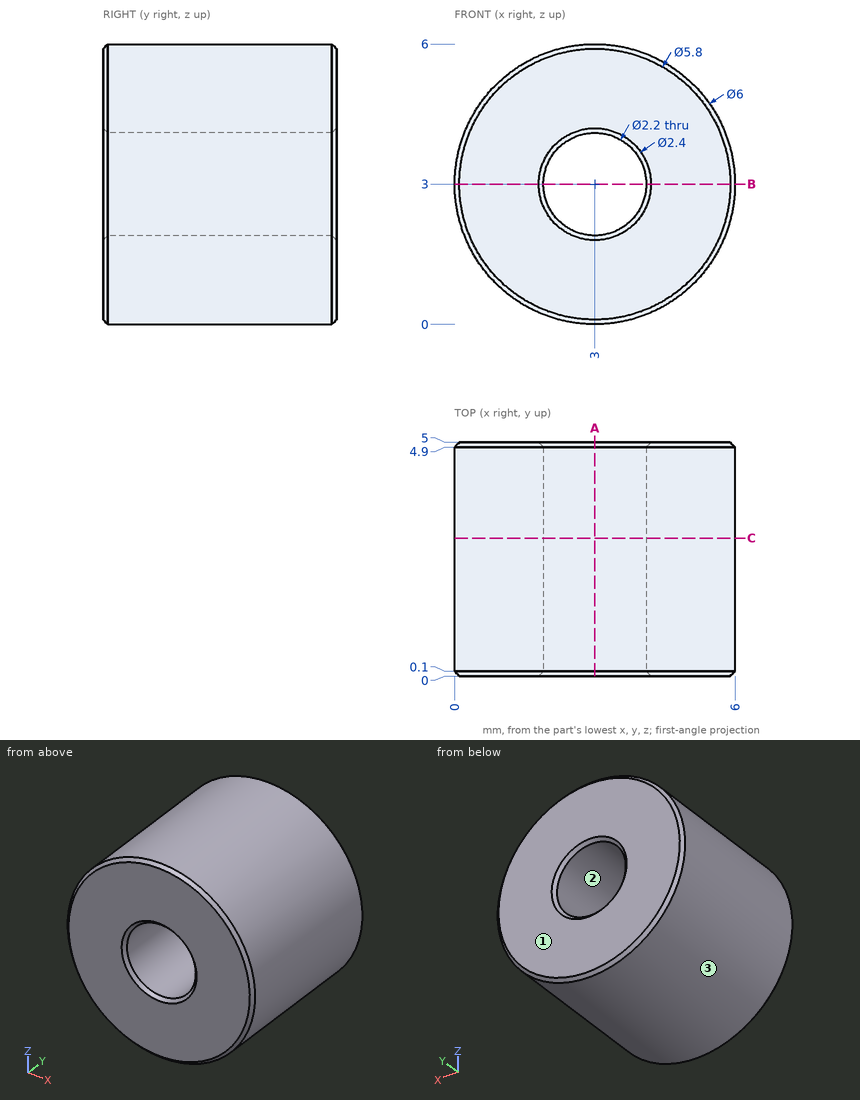
Study the drawing (mm; zero at the part's minimum x, y, z) and answer. Coordinates: 2 decimals unless noted, no trailing zeros. Write each loop counter-clockwise with the first axis right and the second up, starting at its lowest first coordinate (ties: lowest second). Pieces come first, ordered by that corner, then holes. Notation, with made-up numbers: M -4.5,-38 L 7.5,-38 A15 cw 7.5,-19 Z; hole C 1,88 d11. An arc over 180 degrees is marked long. Use a Markdown table: item, result. Add a question column.
1. Given P1, Ø1.5, axis at y = 2.5, z = 5.5, coming from the +X side, flat-ended and moving along its own axis, determine where the tip first touches the part or whether it passes through.
2. Straight lines are drawn through the part: line 1 along X through (y, z) = (1.5, 3); line 2 along X through (y, z) = (0.95, 2.2); line 3 along Z through (x, y) = (3.2, 1.4). For each, find the intervals that lie inside material, in ascending order. Write a range as [from, to].
3. Section B-B (z = 3) is taken. Give the vertices of the cut face in (x, y).
4. Section A-A (x = 3) is taken. Give the vertices of the cut face in (y, z), plus the area to 3 significant figures.
5. Section C-C (y = 2.95) is taken. Give the vertices of the cut face in (x, z), plus the area to 3 significant figures.
6. For a pull along Z with two mould halves and no side action, classify the marked faces 1, 2 and 3 as +Z half, -Z half, draft (parallel to the pull), parting line (faces both ways), or undercut.
Data:
| question | item | result |
|---|---|---|
| 1 | P1 | stops at x = 5.44 |
| 2 | line 1 | x = [0, 1.9], [4.1, 6] |
| 2 | line 2 | x = [0.11, 2.25], [3.75, 5.89] |
| 2 | line 3 | z = [0.01, 1.92], [4.08, 5.99] |
| 3 | outline | M 0,0.1 L 0.1,0 L 1.8,0 L 1.9,0.1 L 1.9,4.9 L 1.8,5 L 0.1,5 L 0,4.9 Z; M 4.1,0.1 L 4.2,0 L 5.9,0 L 6,0.1 L 6,4.9 L 5.9,5 L 4.2,5 L 4.1,4.9 Z |
| 4 | outline | M 0,0.1 L 0.1,0 L 4.9,0 L 5,0.1 L 5,1.8 L 4.9,1.9 L 0.1,1.9 L 0,1.8 Z; M 0,4.2 L 0.1,4.1 L 4.9,4.1 L 5,4.2 L 5,5.9 L 4.9,6 L 0.1,6 L 0,5.9 Z |
| 4 | area | 19.0 mm2 |
| 5 | outline | C 3,3 d6; hole C 3,3 d2.2 |
| 5 | area | 24.5 mm2 |
| 6 | face 1 | draft |
| 6 | face 2 | undercut |
| 6 | face 3 | parting line |
